Autodesk Inventor part; units mm, degrees
ref_plane "YZ Plane" through (0, 0, 0) normal (1, 0, 0) x (0, 1, 0)
ref_plane "XZ Plane" through (0, 0, 0) normal (0, 1, 0) x (-1, 0, 0)
ref_plane "XY Plane" through (0, 0, 0) normal (0, 0, 1) x (1, 0, 0)
sketch "スケッチ1" plane through (0, 0, 0) normal (0, 0, 1) x (1, 0, 0)
  line L0 (-5.5, 3.25) -> (3.5, 3.25)
  line L1 (3.5, 3.25) -> (3.5, -3.25)
  line L2 (3.5, -3.25) -> (-5.5, -3.25)
  line L3 (-5.5, -3.25) -> (-5.5, 3.25)
  line L4 (-5.5, 3.25) -> (3.5, -3.25) construction
  line L5 (3.5, 3.25) -> (-5.5, -3.25) construction
  circle A0 centre (0, 0) radius 2.575
  point P0 (-1, 0)
  point P1 (-1, 0)
  dimension "d0" = 5.15
  dimension "d1" = 9
  dimension "d2" = 3.5
  dimension "d3" = 6.5
extrude "押し出し1" add sketch "スケッチ1" against normal blind 13
sketch "スケッチ2" plane through (-5.5, -3.25, 0) normal (0, -1, 0) x (1, 0, 0)
  circle A0 centre (7, -5) radius 0.75
  circle A1 centre (2, -5) radius 0.75
  line L0 (9, 0) -> (0, 0)
  point P0 (5.5, 0)
  dimension "d6" = 1.5
  dimension "d7" = 5
  dimension "d8" = 1.5
  dimension "d9" = 3.5
extrude "押し出し2" add sketch "スケッチ2" along normal blind 1
sketch "スケッチ3" plane through (-5.5, -3.25, 0) normal (0, -1, 0) x (1, 0, 0)
  line L0 (4.15, -10.75) -> (6.85, -10.75)
  line L1 (6.85, -10.75) -> (6.85, -12.25)
  line L2 (6.85, -12.25) -> (4.15, -12.25)
  line L3 (4.15, -12.25) -> (4.15, -10.75)
  line L4 (4.15, -10.75) -> (6.85, -12.25) construction
  line L5 (6.85, -10.75) -> (4.15, -12.25) construction
  circle A0 centre (7, -5) radius 0.75
  line L6 (1.7, -11.3) -> (2.5, -11.3)
  line L7 (2.5, -11.3) -> (2.5, -13.3)
  line L8 (2.5, -13.3) -> (1.7, -13.3)
  line L9 (1.7, -13.3) -> (1.7, -11.3)
  line L10 (1.7, -11.3) -> (2.5, -13.3) construction
  line L11 (2.5, -11.3) -> (1.7, -13.3) construction
  line L12 (0.2, -7.8) -> (1, -7.8)
  line L13 (1, -7.8) -> (1, -9.8)
  line L14 (1, -9.8) -> (0.2, -9.8)
  line L15 (0.2, -9.8) -> (0.2, -7.8)
  line L16 (0.2, -7.8) -> (1, -9.8) construction
  line L17 (1, -7.8) -> (0.2, -9.8) construction
  circle A1 centre (2, -5) radius 0.75
  point P0 (5.5, 0)
  point P1 (5.5, -11.5)
  point P2 (5.5, -11.5)
  point P3 (2.1, -12.3)
  point P4 (0.6, -8.8)
  dimension "d12" = 1.5
  dimension "d13" = 2.7
  dimension "d15" = 6.5
  dimension "d16" = 0.8
  dimension "d17" = 2
  dimension "d18" = 4.9
  dimension "d19" = 3.8
  dimension "d20" = 3.4
  dimension "d21" = 7.3
extrude "押し出し3" add sketch "スケッチ3" along normal blind 3 contours L0 L1 L2 L3 | L6 L7 L8 L9 | L12 L13 L14 L15
sketch "スケッチ4" plane through (0, 0, -13) normal (0, 0, -1) x (-1, 0, 0)
  line L0 (-3.5, 3.25) -> (-3.5, -3.25)
  line L1 (5.5, -3.25) -> (5.5, 3.25)
  line L2 (-3.5, 3.25) -> (5.5, 3.25)
  line L3 (5.5, 3.25) -> (5.5, -3.25)
  line L4 (5.5, -3.25) -> (-3.5, -3.25)
  line L5 (-3.5, -3.25) -> (-3.5, 3.25)
  point P0 (0, 0)
extrude "押し出し4" add sketch "スケッチ4" against normal blind 3
properties part number "Circuit_HEC3110-01-010"
Work out the finished part from the listing and answer in its coordinate system (mm). A direction names the side the tool comes from. Coordinates: 2 decimals unless noted, no trailing zeros. Loops run counter-clockwise (first coordinate to the right, second up) from the corner with the lowest first, then second, coordinate; pieces in that order, holes last. Notation, with made-up numbers: (-33.75, -15.5) -> (-0.75, -15.5) arc R25 ccw to (-0.75, -3.5) -> close; hole circle Ø5 at (83.25, 22). An arc over 180 degrees is marked (long way). Write each question's results on one line, items separated by ' | '. Start each with the question number.
1) Consider line 1 along Y through (x, z) = (0, -5.75) (3 decimals); line 2 along Z through (x, y) = (-3.5, -4); line 3 along Z through (x, y) = (-0.5, -2). Determine where each line is inside the solid, lowest interval first.
2) The mould has two halves that part along Z. Classify faces 1 (the flat face through (-3, 0, 0)), 2 (the cylindrical face through (-4.095, -3.743, -4.544)), 3 (the flat face through (-1, 3.25, -6)), 4 (the flat face through (0, -5, -12.25)): pulls with the +Z half, pulls with the -Z half, needs draft (parallel to the pull), parting line crosses it, or undercut.
3) For faces 5 (the flat face through (0, 0, -10)), 6 (the cylindrical face through (1.337, -3.743, -4.268)), 7 (the flat face through (-1.35, -5, -12)), 8 (the flat face through (-3, -5, -12)), 9 (the flat face through (1, -4.25, -5)), determine the directions among +Z, -Z, +X, -X, +Y, -Y from which every point of the face is accessible in a straight line to the end or side of a thin tool.
4) Find section B-B on x = -3.5. Determine the outline of the cut face in (y, z), then the cut area to 3 significant figures.
5) Find section C-C on z = -7. Determine the outline of the cut face in (x, y) (3 decimals), then the cut area to 3 significant figures.
6) Find section D-D on y = -1.75. Determine the outline of the cut face in (x, z).
7) Find section A-A on y = -3.75. Determine the outline of the cut face in (x, z).
8) Flat-ended cylindrical pins translate along their axes: P1, Ø1.2, axis at y = -5.5, z = -11.5, coming from the -X side; P2, Ø1, axis at y = -5, z = -8.5, coming from the +X side; P3, Ø1, axis at x = 0.5, y = -2, coming from the -Z side. Find the tip coordinate at first contact, or state that the pin passes through.
Response values:
1) line 1: y = -3.25 to -2.575, 2.575 to 3.25 | line 2: z = -13.3 to -11.3, -5.75 to -4.25 | line 3: z = -13 to -10
2) face 1: pulls with the +Z half | face 2: undercut | face 3: needs draft | face 4: pulls with the -Z half
3) face 5: +Z | face 6: -Y | face 7: +Z, -Z, -Y | face 8: -Z, -Y | face 9: +Z, +X, -X, -Y
4) outline: (-6.25, -13.3) -> (-3.25, -13.3) -> (-3.25, -13) -> (3.25, -13) -> (3.25, 0) -> (-3.25, 0) -> (-3.25, -4.25) -> (-4.25, -4.25) -> (-4.25, -5.75) -> (-3.25, -5.75) -> (-3.25, -11.3) -> (-6.25, -11.3) -> close | area: 92.0 mm^2
5) outline: (-5.5, -3.25) -> (3.5, -3.25) -> (3.5, 3.25) -> (-5.5, 3.25) -> close; hole circle Ø5.15 at (0, 0) | area: 37.7 mm^2
6) outline: (-5.5, -13) -> (3.5, -13) -> (3.5, 0) -> (1.89, 0) -> (1.89, -10) -> (-1.89, -10) -> (-1.89, 0) -> (-5.5, 0) -> close
7) outline: (-5.3, -9.8) -> (-4.5, -9.8) -> (-4.5, -7.8) -> (-5.3, -7.8) -> close; circle Ø1.5 at (-3.5, -5); (-3.8, -13.3) -> (-3, -13.3) -> (-3, -11.3) -> (-3.8, -11.3) -> close; (-1.35, -12.25) -> (1.35, -12.25) -> (1.35, -10.75) -> (-1.35, -10.75) -> close; circle Ø1.5 at (1.5, -5)
8) P1: stops at x = -3.8 | P2: stops at x = -4.5 | P3: stops at z = -13
